```python
from build123d import *

# Parameters (mm, degrees)
CROQUIS1_W              = 500
CROQUIS1_H              = 550
SALIENTE_EXTRUIR1_DEPTH = 50
CROQUIS2_W              = 50
CROQUIS2_H              = 50
CORTAR_EXTRUIR1_DEPTH   = 50
MATRIZL1_COUNT          = 2
MATRIZL1_PITCH          = 500


with BuildPart() as part:
    # Croquis1 → Saliente-Extruir1 (new body)
    with BuildSketch(Plane(origin=(0, 0, 0), x_dir=(1, 0, 0), z_dir=(0, 1, 0))):
        Rectangle(CROQUIS1_W, CROQUIS1_H)
    extrude(amount=SALIENTE_EXTRUIR1_DEPTH)

    # Croquis2 → Cortar-Extruir1 (cut)
    with BuildSketch(Plane(origin=(0, 50, 0), x_dir=(1, 0, 0), z_dir=(0, 1, 0))):
        with Locations((-225, 250)):
            Rectangle(CROQUIS2_W, CROQUIS2_H)
    cortar_extruir1 = extrude(amount=-CORTAR_EXTRUIR1_DEPTH, mode=Mode.SUBTRACT)

    # MatrizL1: Cortar-Extruir1 ×2
    with Locations(*[(0, 0, i * MATRIZL1_PITCH) for i in range(1, MATRIZL1_COUNT)]):
        add(cortar_extruir1, mode=Mode.SUBTRACT)


solid = part.part
```
Can you work these out from the model? Positions are in its coordinate system, mm. A direction names the side the tool comes from. Round coordinates to 2 decimals unless told otherwise and drop trailing zeros. Order: outer loops, then holes, each group sorted by start corner. A loop starts at its lowest first (then second) coordinate and runs counter-clockwise, first axis right, second up.
(1) I'm going to push a flat-ended pin straight in: pin 1 (25 mm diameter, centred on x = -216, y = 33.5, fed in from -Z). Where does the tip first touch, or does it pass through?
Results are:
pin 1: stops at z = -225
(2) If we section it at B-B (x = -206.5): Please give me the cut outline in (y, z), plus the area to 3 significant figures.
Results are:
outline: (0, -225) - (50, -225) - (50, 225) - (0, 225) - close
area: 22,500 mm2
(3) On a 3-axis mill with a long thin cutter (end or side, diameter ignored), from which of +Z, -Z, +X, -X, +Y, -Y can I reach the whole of each face in a straight line? I mean faces 1 (the face through (-250, 25, 3)), 2 (the face through (-200, 25, -250)), 3 (the face through (-225, 25, 225)). Say none if no direction works.
Results are:
face 1: +Z, -Z, -X, +Y, -Y
face 2: -Z, -X, +Y, -Y
face 3: +Z, -X, +Y, -Y
(4) If we section it at A-A (y = 19): Please give me the cut outline in (x, z).
Results are:
outline: (-250, -225) - (-200, -225) - (-200, -275) - (250, -275) - (250, 275) - (-200, 275) - (-200, 225) - (-250, 225) - close
(5) We'd pull the mould along Y, two halves only. Please class faces 4 (the face through (-3, 0, -4)), 5 (the face through (-225, 25, -225)), 6 (the face through (-3, 50, -4)): +Y half, -Y half, draft (parallel to the pull), parting line (faces both ways), or undercut.
Results are:
face 4: -Y half
face 5: draft
face 6: +Y half
(6) If I drill on L1, parallel to X at y = 21, z = 227, over which ranges is the centre line in solid material (lowest first)?
Results are:
L1: x = -200 to 250
